Check sheet for the modelled part. Datum: model origin and axes. Units: mm. Round coordinates to 2 decimals unless told otherwise and drop trailing zeros. Write each loop counter-clockwise with the first axis right and the second up, starting at its lowest first coordinate (ties: lowest second). Pieces come first, ordered by that corner, then holes. Notation, with made-up numbers: (-20.5, -1.5) -> (-12.5, -1.5) arc R12 cw to (-12.5, 4.5) -> close; hole circle Ø10 at (-6, 68). An arc over 180 degrees is marked (long way). Write item = value, one per line.
from build123d import *

# Parameters (mm, degrees)
F0_W      = 145
F0_H      = 126.5
F1_DEPTH  = 3
F2_R      = 1.5
F3_DEPTH  = 3.001
F4_R      = 1.6
F5_DEPTH  = 3.001
F7_R      = 1.6
F8_DEPTH  = 3.001
F9_R      = 1.6
F10_DEPTH = 3.001
F11_R     = 4
F11_R_2   = 1.5
F12_DEPTH = 3.001
F13_DEPTH = 3.001
F15_DEPTH = 3.001
F17_DEPTH = 3.001


with BuildPart() as f1:
    # F0 (on Top) → F1 (new body)
    with BuildSketch(Plane.XY):
        with Locations((72.5, 63.25)):
            Rectangle(F0_W, F0_H)
    extrude(amount=F1_DEPTH)

    # F2 (on face) → F3 (cut, through all)
    with BuildSketch(Plane.XY.offset(3)):
        with Locations((15, 105)):
            Circle(F2_R)
        with Locations((20, 105)):
            Circle(F2_R)
        with Locations((100, 105)):
            Circle(F2_R)
        with Locations((105, 105)):
            Circle(F2_R)
        with Locations((15, 85)):
            Circle(F2_R)
        with Locations((20, 85)):
            Circle(F2_R)
        with Locations((15, 65)):
            Circle(F2_R)
        with Locations((20, 65)):
            Circle(F2_R)
        with Locations((15, 45)):
            Circle(F2_R)
        with Locations((20, 45)):
            Circle(F2_R)
        with Locations((100, 85)):
            Circle(F2_R)
        with Locations((105, 85)):
            Circle(F2_R)
        with Locations((100, 65)):
            Circle(F2_R)
        with Locations((105, 65)):
            Circle(F2_R)
        with Locations((100, 45)):
            Circle(F2_R)
        with Locations((105, 45)):
            Circle(F2_R)
    extrude(amount=-F3_DEPTH, mode=Mode.SUBTRACT)

    # F4 (on face) → F5 (cut, through all)
    with BuildSketch(Plane.XY.offset(3)):
        with Locations((27.5, 105)):
            Circle(F4_R)
        with Locations((67.5, 105)):
            Circle(F4_R)
        with Locations((27.5, 85)):
            Circle(F4_R)
        with Locations((67.5, 85)):
            Circle(F4_R)
        with Locations((27.5, 65)):
            Circle(F4_R)
        with Locations((67.5, 65)):
            Circle(F4_R)
        with Locations((27.5, 45)):
            Circle(F4_R)
        with Locations((67.5, 45)):
            Circle(F4_R)
        with Locations((52.5, 105)):
            Circle(F4_R)
        with Locations((92.5, 105)):
            Circle(F4_R)
        with Locations((52.5, 85)):
            Circle(F4_R)
        with Locations((92.5, 85)):
            Circle(F4_R)
        with Locations((52.5, 65)):
            Circle(F4_R)
        with Locations((92.5, 65)):
            Circle(F4_R)
        with Locations((52.5, 45)):
            Circle(F4_R)
        with Locations((92.5, 45)):
            Circle(F4_R)
    extrude(amount=-F5_DEPTH, mode=Mode.SUBTRACT)

    # F7 (on face) → F8 (cut, through all)
    with BuildSketch(Plane.XY.offset(3)):
        with Locations((125, 106.75)):
            Circle(F7_R)
        with Locations((125, 43.25)):
            Circle(F7_R)
    extrude(amount=-F8_DEPTH, mode=Mode.SUBTRACT)

    # F9 (on face) → F10 (cut, through all)
    with BuildSketch(Plane.XY.offset(3)):
        with Locations((36.45, 25)):
            Circle(F9_R)
        with Locations((83.55, 25)):
            Circle(F9_R)
    extrude(amount=-F10_DEPTH, mode=Mode.SUBTRACT)

    # F11 (on face) → F12 (cut, through all)
    with BuildSketch(Plane.XY.offset(3)):
        with Locations((105, 15)):
            Circle(F11_R)
        with Locations((125, 15)):
            Circle(F11_R)
        with Locations((105, 25)):
            Circle(F11_R_2)
        with Locations((125, 25)):
            Circle(F11_R_2)
    extrude(amount=-F12_DEPTH, mode=Mode.SUBTRACT)

    # F6 (on face) → F13 (cut, through all)
    with BuildSketch(Plane.XY.offset(3)):
        with BuildLine():
            Line((48, 110.5), (32, 110.5))
            ThreePointArc((32, 110.5), (30.467911, 109.785575), (30.030384, 108.152704))
            Line((30.030384, 108.152704), (31.264673, 101.152704))
            ThreePointArc((31.264673, 101.152704), (31.948714, 99.967911), (33.234289, 99.5))
            Line((33.234289, 99.5), (46.765711, 99.5))
            ThreePointArc((46.765711, 99.5), (48.051286, 99.967911), (48.735327, 101.152704))
            Line((48.735327, 101.152704), (49.969616, 108.152704))
            ThreePointArc((49.969616, 108.152704), (49.532089, 109.785575), (48, 110.5))
        make_face()
        with BuildLine():
            Line((88, 110.5), (72, 110.5))
            ThreePointArc((72, 110.5), (70.467911, 109.785575), (70.030384, 108.152704))
            Line((70.030384, 108.152704), (71.264673, 101.152704))
            ThreePointArc((71.264673, 101.152704), (71.948714, 99.967911), (73.234289, 99.5))
            Line((73.234289, 99.5), (86.765711, 99.5))
            ThreePointArc((86.765711, 99.5), (88.051286, 99.967911), (88.735327, 101.152704))
            Line((88.735327, 101.152704), (89.969616, 108.152704))
            ThreePointArc((89.969616, 108.152704), (89.532089, 109.785575), (88, 110.5))
        make_face()
        with BuildLine():
            Line((48, 90.5), (32, 90.5))
            ThreePointArc((32, 90.5), (30.467911, 89.785575), (30.030384, 88.152704))
            Line((30.030384, 88.152704), (31.264673, 81.152704))
            ThreePointArc((31.264673, 81.152704), (31.948714, 79.967911), (33.234289, 79.5))
            Line((33.234289, 79.5), (46.765711, 79.5))
            ThreePointArc((46.765711, 79.5), (48.051286, 79.967911), (48.735327, 81.152704))
            Line((48.735327, 81.152704), (49.969616, 88.152704))
            ThreePointArc((49.969616, 88.152704), (49.532089, 89.785575), (48, 90.5))
        make_face()
        with BuildLine():
            Line((88, 90.5), (72, 90.5))
            ThreePointArc((72, 90.5), (70.467911, 89.785575), (70.030384, 88.152704))
            Line((70.030384, 88.152704), (71.264673, 81.152704))
            ThreePointArc((71.264673, 81.152704), (71.948714, 79.967911), (73.234289, 79.5))
            Line((73.234289, 79.5), (86.765711, 79.5))
            ThreePointArc((86.765711, 79.5), (88.051286, 79.967911), (88.735327, 81.152704))
            Line((88.735327, 81.152704), (89.969616, 88.152704))
            ThreePointArc((89.969616, 88.152704), (89.532089, 89.785575), (88, 90.5))
        make_face()
        with BuildLine():
            Line((48, 70.5), (32, 70.5))
            ThreePointArc((32, 70.5), (30.467911, 69.785575), (30.030384, 68.152704))
            Line((30.030384, 68.152704), (31.264673, 61.152704))
            ThreePointArc((31.264673, 61.152704), (31.948714, 59.967911), (33.234289, 59.5))
            Line((33.234289, 59.5), (46.765711, 59.5))
            ThreePointArc((46.765711, 59.5), (48.051286, 59.967911), (48.735327, 61.152704))
            Line((48.735327, 61.152704), (49.969616, 68.152704))
            ThreePointArc((49.969616, 68.152704), (49.532089, 69.785575), (48, 70.5))
        make_face()
        with BuildLine():
            Line((88, 70.5), (72, 70.5))
            ThreePointArc((72, 70.5), (70.467911, 69.785575), (70.030384, 68.152704))
            Line((70.030384, 68.152704), (71.264673, 61.152704))
            ThreePointArc((71.264673, 61.152704), (71.948714, 59.967911), (73.234289, 59.5))
            Line((73.234289, 59.5), (86.765711, 59.5))
            ThreePointArc((86.765711, 59.5), (88.051286, 59.967911), (88.735327, 61.152704))
            Line((88.735327, 61.152704), (89.969616, 68.152704))
            ThreePointArc((89.969616, 68.152704), (89.532089, 69.785575), (88, 70.5))
        make_face()
        with BuildLine():
            Line((48, 50.5), (32, 50.5))
            ThreePointArc((32, 50.5), (30.467911, 49.785575), (30.030384, 48.152704))
            Line((30.030384, 48.152704), (31.264673, 41.152704))
            ThreePointArc((31.264673, 41.152704), (31.948714, 39.967911), (33.234289, 39.5))
            Line((33.234289, 39.5), (46.765711, 39.5))
            ThreePointArc((46.765711, 39.5), (48.051286, 39.967911), (48.735327, 41.152704))
            Line((48.735327, 41.152704), (49.969616, 48.152704))
            ThreePointArc((49.969616, 48.152704), (49.532089, 49.785575), (48, 50.5))
        make_face()
        with BuildLine():
            Line((88, 50.5), (72, 50.5))
            ThreePointArc((72, 50.5), (70.467911, 49.785575), (70.030384, 48.152704))
            Line((70.030384, 48.152704), (71.264673, 41.152704))
            ThreePointArc((71.264673, 41.152704), (71.948714, 39.967911), (73.234289, 39.5))
            Line((73.234289, 39.5), (86.765711, 39.5))
            ThreePointArc((86.765711, 39.5), (88.051286, 39.967911), (88.735327, 41.152704))
            Line((88.735327, 41.152704), (89.969616, 48.152704))
            ThreePointArc((89.969616, 48.152704), (89.532089, 49.785575), (88, 50.5))
        make_face()
    extrude(amount=-F13_DEPTH, mode=Mode.SUBTRACT)

    # F14 (on face) → F15 (cut, through all)
    with BuildSketch(Plane.XY.offset(3)):
        with BuildLine():
            ThreePointArc((121.847296, 104.3), (120.214425, 103.862473), (119.5, 102.330384))
            Line((119.5, 102.330384), (119.5, 47.669616))
            ThreePointArc((119.5, 47.669616), (120.214425, 46.137527), (121.847296, 45.7))
            Line((121.847296, 45.7), (128.847296, 46.934289))
            ThreePointArc((128.847296, 46.934289), (130.032089, 47.618329), (130.5, 48.903904))
            Line((130.5, 48.903904), (130.5, 101.096096))
            ThreePointArc((130.5, 101.096096), (130.032089, 102.381671), (128.847296, 103.065711))
            Line((128.847296, 103.065711), (121.847296, 104.3))
        make_face()
    extrude(amount=-F15_DEPTH, mode=Mode.SUBTRACT)

    # F16 (on face) → F17 (cut, through all)
    with BuildSketch(Plane.XY.offset(3)):
        with BuildLine():
            Line((79.030384, 30.5), (40.969616, 30.5))
            ThreePointArc((40.969616, 30.5), (39.437527, 29.785575), (39, 28.152704))
            Line((39, 28.152704), (40.234289, 21.152704))
            ThreePointArc((40.234289, 21.152704), (40.918329, 19.967911), (42.203904, 19.5))
            Line((42.203904, 19.5), (77.796096, 19.5))
            ThreePointArc((77.796096, 19.5), (79.081671, 19.967911), (79.765711, 21.152704))
            Line((79.765711, 21.152704), (81, 28.152704))
            ThreePointArc((81, 28.152704), (80.562473, 29.785575), (79.030384, 30.5))
        make_face()
    extrude(amount=-F17_DEPTH, mode=Mode.SUBTRACT)


solid = f1.part
(1) Go/stop test with a flat-tipped pin: P1, Ø1.9, axis at x = 52.5, y = 45, coming from the +Z side. Record where the tip stops, or that it passes through.
Worked answers:
P1 = through
(2) Sectioned sample at D-D on y = 73. Enter the section's corners in (x, z), then the cut area to 3 significant figures.
Worked answers:
outline = (0, 0) -> (119.5, 0) -> (119.5, 3) -> (0, 3) -> close; (130.5, 0) -> (145, 0) -> (145, 3) -> (130.5, 3) -> close
area = 402 mm²
(3) Sectioned sample at C-C on x = 92.5. Enter the section's corners in (y, z).
Worked answers:
outline = (0, 0) -> (43.4, 0) -> (43.4, 3) -> (0, 3) -> close; (46.6, 0) -> (63.4, 0) -> (63.4, 3) -> (46.6, 3) -> close; (66.6, 0) -> (83.4, 0) -> (83.4, 3) -> (66.6, 3) -> close; (86.6, 0) -> (103.4, 0) -> (103.4, 3) -> (86.6, 3) -> close; (106.6, 0) -> (126.5, 0) -> (126.5, 3) -> (106.6, 3) -> close
(4) Material ranges on L1, parallel to Y at x = 78, z = 2.2; L2, parallel to Y at x = 15, z = 2.2; L3, parallel to Y at x = 83.55, z = 1.05, recorded low to high. Write a range as [from, to].
Worked answers:
L1 = [0, 19.51], [30.5, 39.5], [50.5, 59.5], [70.5, 79.5], [90.5, 99.5], [110.5, 126.5]
L2 = [0, 43.5], [46.5, 63.5], [66.5, 83.5], [86.5, 103.5], [106.5, 126.5]
L3 = [0, 23.4], [26.6, 39.5], [50.5, 59.5], [70.5, 79.5], [90.5, 99.5], [110.5, 126.5]
(5) Sectioned sample at B-B on x = 36.45. Enter the section's corners in (y, z).
Worked answers:
outline = (0, 0) -> (23.4, 0) -> (23.4, 3) -> (0, 3) -> close; (26.6, 0) -> (39.5, 0) -> (39.5, 3) -> (26.6, 3) -> close; (50.5, 0) -> (59.5, 0) -> (59.5, 3) -> (50.5, 3) -> close; (70.5, 0) -> (79.5, 0) -> (79.5, 3) -> (70.5, 3) -> close; (90.5, 0) -> (99.5, 0) -> (99.5, 3) -> (90.5, 3) -> close; (110.5, 0) -> (126.5, 0) -> (126.5, 3) -> (110.5, 3) -> close
(6) Release check for a two-part mould opening along X. For faces 1 (the flat face through (49.344, 44.604, 1.521)), 2 (the flat face through (55, 64, 0)) record: pulls with the +X half, pulls with the -X half, needs draft (parallel to the pull), parting line crosses it, or undercut.
Worked answers:
face_1 = undercut
face_2 = needs draft
(7) Sectioned sample at A-A on y = 15. Enter the section's corners in (x, z), then the cut area to 3 significant figures.
Worked answers:
outline = (0, 0) -> (101, 0) -> (101, 3) -> (0, 3) -> close; (109, 0) -> (121, 0) -> (121, 3) -> (109, 3) -> close; (129, 0) -> (145, 0) -> (145, 3) -> (129, 3) -> close
area = 387 mm²
